```python
from build123d import *

# Parameters (mm, degrees)
F0_R     = 9.525
F1_DEPTH = 1.27
F2_W     = 1.905
F2_H     = 6.35
F3_DEPTH = 25.4
F4_R     = 1.5875
F5_DEPTH = 14.606


with BuildPart() as f1:
    # F0 (on Front) → F1 (new body)
    with BuildSketch(Plane.XZ):
        Circle(F0_R)
    extrude(amount=F1_DEPTH)

    # F2 (on face) → F3 (join)
    with BuildSketch(Plane(origin=(0, 0, 0), x_dir=(-1, 0, 0), z_dir=(0, 1, 0))):
        with Locations((-4.1275, 0)):
            Rectangle(F2_W, F2_H)
        with Locations((4.1275, 0)):
            Rectangle(F2_W, F2_H)
    extrude(amount=F3_DEPTH)

    # F4 (on face) → F5 (cut, through all)
    with BuildSketch(Plane.YZ.offset(5.08)):
        with Locations((20.32, 0)):
            Circle(F4_R)
    extrude(amount=-F5_DEPTH, mode=Mode.SUBTRACT)


solid = f1.part
```
Design review of the part built by this model. Coordinates are the model's own, in mm. A direction names the side the tool comes from. Coordinates: 2 decimals unless noted, no trailing zeros. Order: outer loops, then holes, each group sorted by start corner. A loop starts at its lowest first (then second) coordinate and runs counter-clockwise, first axis right, second up. Notation, with made-up numbers: M 18.5,82 L 55.5,82 A17 ccw 55.5,98 Z; hole C -8.5,74 d9. An arc over 180 degrees is marked long. Answer as a JSON object with one key per item and string values. Group by question number.
1) Add section A-A, the plane y = 18.25. Write out the cut boundary in (x, z) (3 decimals), then the cut area to 3 significant figures.
2) Add section C-C, the plane x = 4.25. Write out the cut boundary in (y, z) (1 decimal).
3) Add section D-D, the plane x = 0. Write out the cut boundary in (y, z) (3 decimals), then the cut area to 3 significant figures.
4) Mouldability with a two-part tool opening along X and no side actions: class faces 1 (the flat face through (-4, 13, -3.175)), 2 (the flat face through (3.175, 13, 0)), 3 (the flat face through (0, 0, 0)), 4 (the flat face through (-5.08, 13, 0)) as pulls with the +X half, pulls with the -X half, needs draft (parallel to the pull), parting line crosses it, or undercut.
5) Wall thickness on L1, parallel to X at y = 2, z = 0 (3 decimals); L2, parallel to Z at x = -4.15, y = 20.32 (1 decimal); L3, parallel to Y at x = -0.5, z = -5.5: over which ranges is each line inside the solid? List them lowest first.
6) Tool access review of faces 5 (the flat face through (4, 13, -3.175)), 6 (the flat face through (4, 13, 3.175)), 7 (the flat face through (-3.175, 13, 0)): name each direction out of +Z, -Z, +X, -X, +Y, -Y from which nothing blocks a thin tool from reaching the whole face with its end or side.
7) Add section B-B, the plane z = 0. Write out the cut boundary in (x, y) (1 decimal).
8) For pin 1 (3 mm diameter, centred on y = 16, z = -1, fed in from -X); pin 2 (5 mm diameter, centred on x = 0, z = -5, fed in from +Y); pin 3 (10 mm diameter, centred on y = 17, z = -4, fed in from +X), all flat-tipped, find the tip position at first contact; note any pin that passes through.
Computed values:
{
 "1": {"outline": "M -5.08,-3.175 L -3.175,-3.175 L -3.175,3.175 L -5.08,3.175 Z; M 3.175,-3.175 L 5.08,-3.175 L 5.08,3.175 L 3.175,3.175 Z", "area": "24.2 mm^2"},
 "2": {"outline": "M -1.3,-8.5 L 0,-8.5 L 0,-3.2 L 25.4,-3.2 L 25.4,3.2 L 0,3.2 L 0,8.5 L -1.3,8.5 Z; hole C 20.3,0 d3.2"},
 "3": {"outline": "M -1.27,-9.525 L 0,-9.525 L 0,9.525 L -1.27,9.525 Z", "area": "24.2 mm^2"},
 "4": {"face 1": "needs draft", "face 2": "undercut", "face 3": "undercut", "face 4": "pulls with the -X half"},
 "5": {"L1": "x = -5.08 to -3.175, 3.175 to 5.08", "L2": "z = -3.2 to -1.6, 1.6 to 3.2", "L3": "y = -1.27 to 0"},
 "6": {"face 5": "-Z, +X, -X, +Y", "face 6": "+Z, +X, -X, +Y", "face 7": "+Z, -Z, +Y"},
 "7": {"outline": "M -9.5,-1.3 L 9.5,-1.3 L 9.5,0 L 5.1,0 L 5.1,18.7 L 3.2,18.7 L 3.2,0 L -3.2,0 L -3.2,18.7 L -5.1,18.7 L -5.1,0 L -9.5,0 Z; M -5.1,21.9 L -3.2,21.9 L -3.2,25.4 L -5.1,25.4 Z; M 3.2,21.9 L 5.1,21.9 L 5.1,25.4 L 3.2,25.4 Z"},
 "8": {"pin 1": "stops at x = -5.08", "pin 2": "stops at y = 0", "pin 3": "stops at x = 5.08"}
}
